Study the drawing (mm; zero at the part's minimum x, y, z) and answer. Give positions to 0.01 mm unless a question says otherwise; leave off trailing zeros. Order: outer loops, then holes, each group sorted by start corner. A loop starts at its lowest first (then second) coordinate and runs counter-clockwise, first axis right, second up. Notation, with made-up numbers: (88, -27.5) - (116, -27.5) arc R33 ccw to (116, 9.5) - close; hole circle Ø3 at (-18.5, 26). An arc over 180 degrees is marked (long way). Return JSON: item names as keys, results as strings.
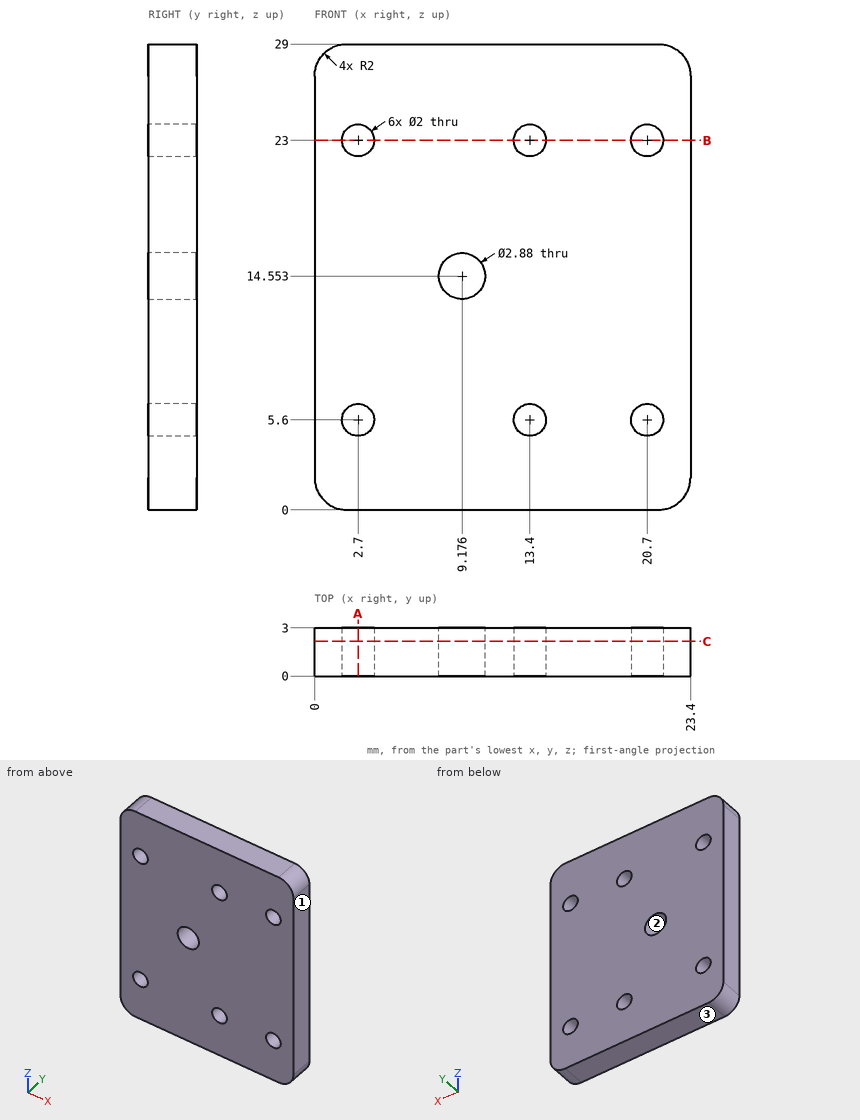
Q1. A cutting plane is placed at B-B (z = 23). Write down the section's boundary in (x, y).
Values:
{"outline": "(0, 0) - (1.7, 0) - (1.7, 3) - (0, 3) - close; (3.7, 0) - (12.4, 0) - (12.4, 3) - (3.7, 3) - close; (14.4, 0) - (19.7, 0) - (19.7, 3) - (14.4, 3) - close; (21.7, 0) - (23.4, 0) - (23.4, 3) - (21.7, 3) - close"}
Q2. Consider L1, parallel to X at y = 0.75, z = 5.6; L2, parallel to X at y = 2.65, z = 14.5 (3 decimals); L3, parallel to Z at x = 13.75, y = 2.55. Determine where each line is inside the solid, lowest interval first.
Values:
{"L1": "x = 0 to 1.7, 3.7 to 12.4, 14.4 to 19.7, 21.7 to 23.4", "L2": "x = 0 to 7.737, 10.615 to 23.4", "L3": "z = 0 to 4.66, 6.54 to 22.06, 23.94 to 29"}
Q3. A cutting plane is placed at A-A (x = 2.7). Write down the section's boundary in (y, z), and give its area (3 significant figures).
Values:
{"outline": "(0, 0) - (3, 0) - (3, 4.6) - (0, 4.6) - close; (0, 6.6) - (3, 6.6) - (3, 22) - (0, 22) - close; (0, 24) - (3, 24) - (3, 29) - (0, 29) - close", "area": "75.0 mm²"}
Q4. Given pin 1 (1 mm diameter, centred on x = 7, y = 1.5, fed in from -Z); pin 2 (1.6 mm diameter, centred on x = 20.7, z = 5.6, fed in from -Y), each flat-ended and moving along its own axis, determine where each tip first touches the part or whether it passes through.
Values:
{"pin 1": "stops at z = 0", "pin 2": "passes through"}
Q5. A cutting plane is placed at C-C (y = 2.15). Write down the section's boundary in (x, z).
Values:
{"outline": "(0, 2) arc R2 ccw to (2, 0) - (21.4, 0) arc R2 ccw to (23.4, 2) - (23.4, 27) arc R2 ccw to (21.4, 29) - (2, 29) arc R2 ccw to (0, 27) - close; hole circle Ø2 at (2.7, 5.6); hole circle Ø2 at (2.7, 23); hole circle Ø2.88 at (9.18, 14.55); hole circle Ø2 at (13.4, 5.6); hole circle Ø2 at (13.4, 23); hole circle Ø2 at (20.7, 5.6); hole circle Ø2 at (20.7, 23)"}
Q6. Determine the mould class of the marked faces 1, 2 and 3 for opening direction X: released by +X, released by -X, zero draft, split by the parting line, or undercut.
Values:
{"face 1": "released by +X", "face 2": "undercut", "face 3": "zero draft"}
